Design review of the part built by this model. Coordinates are the model's own, in mm. A direction names the side the tool comes from. Give positions to 0.01 mm unless a question says otherwise; leave off trailing zeros. Loops run counter-clockwise (first coordinate to the right, second up) from the corner with the lowest first, then second, coordinate; pieces in that order, holes last. Notation, with made-up numbers: M -30.75,85.25 L 12.25,85.25 A29 cw 12.25,112.25 Z; hole C 88,-23 d3. An arc over 180 degrees is marked long. Use CSV: the item, a comma, the result in double quotes.
from build123d import *

# Parameters (mm, degrees)
BOSS_EXTRUDE1_DEPTH = 7
SKETCH2_R           = 1.65
CUT_EXTRUDE1_DEPTH  = 139.646530772
SKETCH3_R           = 1.65
CUT_EXTRUDE2_DEPTH  = 6.35
FILLET1_R           = 3
SKETCH4_R           = 2.25
CUT_EXTRUDE3_DEPTH  = 6.35


with BuildPart() as part:
    # Sketch1 → Boss-Extrude1 (new body)
    with BuildSketch(Plane(origin=(0, 0, 0), x_dir=(1, 0, 0), z_dir=(0, 1, 0))):
        Polygon((0, 0), (53.650408323, 0), (53.650408323, 30.8), (60.000408323, 30.8), (60.000408323, 15.8), (75.000408323, 15.8), (75.000408323, 9.45), (60.000408323, 9.45), (60.000408323, -6.35), (-59.999591677, -6.35), (-60.000408323, 9.45), (-75.000408323, 9.45), (-75.000408323, 15.8), (-60.000408323, 15.8), (-60.000408323, 30.8), (-53.650408323, 30.8), (-53.650408323, 0), align=None)
    extrude(amount=BOSS_EXTRUDE1_DEPTH)

    # Sketch2 → Cut-Extrude1 (cut, through all)
    with BuildSketch(Plane(origin=(60.000408323, 0, 0), x_dir=(0, 0, -1), z_dir=(1, 0, 0))):
        with Locations((23.3, 3.5)):
            Circle(SKETCH2_R)
    extrude(amount=-CUT_EXTRUDE1_DEPTH, mode=Mode.SUBTRACT)

    # Sketch3 → Cut-Extrude2 (cut)
    with BuildSketch(Plane(origin=(0, 0, -15.8), x_dir=(-1, 0, 0), z_dir=(0, 0, -1))):
        with Locations((-67.500408323, 3.5)):
            Circle(SKETCH3_R)
        with Locations((67.500408323, 3.5)):
            Circle(SKETCH3_R)
    extrude(amount=-CUT_EXTRUDE2_DEPTH, mode=Mode.SUBTRACT)

    # Fillet1
    fillet1_edges = [part.edges().sort_by_distance(p)[0] for p in [
        (53.650408323, 3.5, 0),
        (60.000408323, 3.5, -9.45),
        (60.000408323, 3.5, 6.35),
        (-59.999591677, 3.5, 6.35),
        (-60.000408323, 3.5, -9.45),
        (-53.650408323, 3.5, 0),
    ]]
    fillet(fillet1_edges, radius=FILLET1_R)

    # Sketch4 → Cut-Extrude3 (cut)
    with BuildSketch(Plane.XY.offset(6.35)):
        with Locations((5.000165403, 3.5)):
            Circle(SKETCH4_R)
        with Locations((-4.999834586, 3.500472565)):
            Circle(SKETCH4_R)
    extrude(amount=-CUT_EXTRUDE3_DEPTH, mode=Mode.SUBTRACT)


solid = part.part
(1) Clearance check with flat-ended pins moving along their axes: P1, Ø2, axis at y = 4, z = -24.5, coming from the -X side; P2, Ø3, axis at y = 3.5, z = -23.3, coming from the +X side; P3, Ø2, axis at y = 4, z = -20.5, coming from the +X side; P4, Ø2, axis at x = -68, y = 2, coming from the +Z side. State where each tip first meets the part, or that it passes through.
A:
P1,"x = -60"
P2,"through"
P3,"x = 60"
P4,"z = -9.45"
(2) We need section B-B on z = -23.3. State the section outline as (x, y) points.
A:
outline,"M -60,0 L -53.65,0 L -53.65,1.85 L -60,1.85 Z; M -60,5.15 L -53.65,5.15 L -53.65,7 L -60,7 Z; M 53.65,0 L 60,0 L 60,1.85 L 53.65,1.85 Z; M 53.65,5.15 L 60,5.15 L 60,7 L 53.65,7 Z"
(3) Wall thickness on line 1 along X through (y, z) = (3.75, -14); line 2 along X through (y, z) = (6.75, -6); line 3 along X through (y, z) = (0.5, -9.5): over which ranges is each line inside the solid? List them lowest first. Write a range as [from, to].
A:
line 1,"[-75, -69.13], [-65.87, -53.65], [53.65, 65.87], [69.13, 75]"
line 2,"[-60, -53.65], [53.65, 60]"
line 3,"[-75, -53.65], [53.65, 75]"
(4) The part is to be moulded in two halves that separate along Y. For faces 1 (the cylindrical face through (56.87, 3.57, -21.65)), 2 (the flat face through (-60, 3.5, -21.5)), say which applies: released by +Y, released by -Y, zero draft, split by the parting line, or undercut.
A:
face 1,"undercut"
face 2,"zero draft"
(5) We need section D-D on x = 58.5. State the section outline as (y, z) points, then the cut area to 3 significant figures.
A:
outline,"M 0,-30.8 L 7,-30.8 L 7,5.95 L 0,5.95 Z; hole C 3.5,-23.3 d3.3"
area,"249 mm²"
(6) We need section A-A on z = -11. State the section outline as (x, y) points, then the cut area to 3 significant figures.
A:
outline,"M -75,0 L -53.65,0 L -53.65,7 L -75,7 Z; M 53.65,0 L 75,0 L 75,7 L 53.65,7 Z; hole C -67.5,3.5 d3.3; hole C 67.5,3.5 d3.3"
area,"282 mm²"
(7) Machinability: for faces 3 (the flat face through (65.7, 3.5, -15.8)), 4 (the cylindrical face through (59.145, 3.549, 5.448)), 5 (the cylindrical face through (-52.748, 3.549, -0.855)), 6 (the flat face through (-70, 3, -9.45)), 7 (the cylindrical face through (-66.284, 4.615, -12.669)), which of the approach directions +Z, -Z, +X, -X, +Y, -Y give a long, thin tool a straight path to every point of the face, cutting with its end or side? Answer none if there is none.
A:
face 3,"-Z, +X, +Y, -Y"
face 4,"+Z, +X, +Y, -Y"
face 5,"-Z, +Y, -Y"
face 6,"+Z, -X, +Y, -Y"
face 7,"+Z, -Z"
(8) We need section C-C on x = -35. State the section outline as (y, z) points, then the cut area to 4 significant figures.
A:
outline,"M 0,0 L 7,0 L 7,6.35 L 0,6.35 Z"
area,"44.45 mm²"
